CAD build for the part. Positions are in the model's coordinates, mm. A direction names the side the tool comes from. Round coordinates to 2 decimals unless told otherwise and drop trailing zeros. Loops run counter-clockwise (first coordinate to the right, second up) from the corner with the lowest first, then second, coordinate; pieces in that order, holes last. Notation, with made-up numbers: (19.5, 11) -> (40.5, 11) arc R5 ccw to (40.5, 15) -> close; hole circle Ø11 at (19.25, 24.5). An arc over 180 degrees is marked (long way). Answer as CSV lines item,"result".
```python
from build123d import *

# Parameters (mm, degrees)
F0_W     = 6.35
F0_H     = 6.35
F0_W_2   = 495.3
F0_H_2   = 241.3
F1_DEPTH = 127
F2_DEPTH = 6.35
F3_W     = 25.4
F3_H     = 25.4
F4_DEPTH = 25.4
F5_W     = 508
F5_H     = 127
F6_DEPTH = 25.4
F7_W     = 609.6
F7_H     = 127
F8_DEPTH = 12.7
F9_R     = 6.35


with BuildPart() as f1:
    # F0 (on Top) → F1 (new body)
    with BuildSketch(Plane.XY):
        with Locations((-250.825, 123.825)):
            Rectangle(F0_W, F0_H)
        with Locations((-250.825, -123.825)):
            Rectangle(F0_W, F0_H)
        with Locations((250.825, -123.825)):
            Rectangle(F0_W, F0_H)
        with Locations((250.825, 123.825)):
            Rectangle(F0_W, F0_H)
        with Locations((0, 123.825)):
            Rectangle(F0_W_2, F0_H)
        with Locations((0, -123.825)):
            Rectangle(F0_W_2, F0_H)
        with Locations((250.825, 0)):
            Rectangle(F0_W, F0_H_2)
        with Locations((-250.825, 0)):
            Rectangle(F0_W, F0_H_2)
    extrude(amount=F1_DEPTH)

    # F0 (on Top) → F2 (join)
    with BuildSketch(Plane.XY):
        Rectangle(F0_W_2, F0_H_2)
    extrude(amount=F2_DEPTH)

    # F3 (on face) → F4 (join)
    with BuildSketch(Plane.XY.offset(6.35)):
        with Locations((-234.95, -107.95)):
            Rectangle(F3_W, F3_H)
        with Locations((-234.95, 107.95)):
            Rectangle(F3_W, F3_H)
        with Locations((234.95, 107.95)):
            Rectangle(F3_W, F3_H)
        with Locations((234.95, -107.95)):
            Rectangle(F3_W, F3_H)
    extrude(amount=F4_DEPTH)

    # F5 (on face) → F6 (join)
    with BuildSketch(Plane.XZ.offset(127)):
        with Locations((0, 63.5)):
            Rectangle(F5_W, F5_H)
    extrude(amount=F6_DEPTH)

    # F7 (on face) → F8 (join)
    with BuildSketch(Plane.XZ.offset(152.4)):
        with Locations((0, 63.5)):
            Rectangle(F7_W, F7_H)
    extrude(amount=F8_DEPTH)

    # F9
    f9_edges = [f1.edges().sort_by_distance(p)[0] for p in [
        (-304.8, -165.1, 63.5),
        (0, -165.1, 0),
        (304.8, -165.1, 63.5),
        (0, -165.1, 127),
    ]]
    fillet(f9_edges, radius=F9_R)


solid = f1.part
```
Q1. Slice it at A-A, the plane z = 42.5. Give the cut face in (x, y).
Results:
outline,"(-304.8, -158.75) arc R6.35 ccw to (-298.45, -165.1) -> (298.45, -165.1) arc R6.35 ccw to (304.8, -158.75) -> (304.8, -152.4) -> (254, -152.4) -> (254, 127) -> (-254, 127) -> (-254, -152.4) -> (-304.8, -152.4) -> close; hole (-247.65, -120.65) -> (247.65, -120.65) -> (247.65, 120.65) -> (-247.65, 120.65) -> close"
Q2. Slice it at D-D, the plane x = -232. Give the cut face in (y, z).
Results:
outline,"(-165.1, 6.35) arc R6.35 ccw to (-158.75, 0) -> (127, 0) -> (127, 127) -> (120.65, 127) -> (120.65, 31.75) -> (95.25, 31.75) -> (95.25, 6.35) -> (-95.25, 6.35) -> (-95.25, 31.75) -> (-120.65, 31.75) -> (-120.65, 127) -> (-158.75, 127) arc R6.35 ccw to (-165.1, 120.65) -> close"
Q3. Slice it at C-C, the plane x = 46. Give the cut face in (y, z), and give its area (3 significant figures).
Results:
outline,"(-165.1, 6.35) arc R6.35 ccw to (-158.75, 0) -> (127, 0) -> (127, 127) -> (120.65, 127) -> (120.65, 6.35) -> (-120.65, 6.35) -> (-120.65, 127) -> (-158.75, 127) arc R6.35 ccw to (-165.1, 120.65) -> close"
area,"7,970 mm2"
Q4. Tool access for faces 1 (the flat face through (-47, -121, 127)), 2 (the flat face through (-235, 108, 31.75)), 3 (the flat face through (-254, -11, 63)): list every direction of +Z, -Z, +X, -X, +Y, -Y with a clear straight run to the whole face (end or side of a thin tool).
Results:
face 1,"+Z, +X, -X, +Y, -Y"
face 2,"+Z"
face 3,"+Z, -Z, -X, +Y"
Q5. Two-plate mould, pull along Y, no slides. Class faces 4 (the flat face through (-222.25, -108, 19)), 5 (the flat face through (-280, -152.4, 64)), 6 (the flat face through (-4, -14, 0)): pulls with the +Y half, pulls with the -Y half, needs draft (parallel to the pull), parting line crosses it, or undercut.
Results:
face 4,"undercut"
face 5,"pulls with the +Y half"
face 6,"needs draft"
Q6. Drop flat-ended pins along their axis: pin 1 Ø2 at (x, y) = (-58, 66) entering from +Z; pin 2 Ø12.5 at (x, y) = (-234.5, 103.5) entering from +Z; pin 3 Ø12.5 at (y, z) = (105.5, 23.5) entering from +X; pin 4 Ø10 at (x, y) = (-238, 23.5) entering from -Z. Give the stop position or say it passes through.
Results:
pin 1,"z = 6.35"
pin 2,"z = 31.75"
pin 3,"x = 254"
pin 4,"z = 0"
Q7. Probe L1, parallel to Y at x = 6.5, z = 7; L2, parallel to X at y = 51, z = 33.5; L3, parallel to X at y = -110, z = 19. List the from-to ranges inside material, lowest first. Write a range as [from, to].
Results:
L1,"[-165.1, -120.65], [120.65, 127]"
L2,"[-254, -247.65], [247.65, 254]"
L3,"[-254, -222.25], [222.25, 254]"
Q8. Slice it at B-B, the plane y = 82. Give the cut face in (x, z).
Results:
outline,"(-254, 0) -> (254, 0) -> (254, 127) -> (247.65, 127) -> (247.65, 6.35) -> (-247.65, 6.35) -> (-247.65, 127) -> (-254, 127) -> close"
